Geometry check sheet. Reference: the model listing, model coordinates, mm. Face numbers are marked on the shaded views. A direction names the side the tool comes from. Coordinates: 2 decimals unless noted, no trailing zeros. Order: outer loops, then holes, each group sorted by start corner. A loop starts at its lowest first (then second) coordinate and runs counter-clockwise, first axis right, second up. Notation, with made-up numbers: (-29, 18) - (-16, 18) arc R16 ccw to (-16, 27) - close; hole circle Ø11 at (16, -1.5). An arc over 180 degrees is marked (long way). Return JSON: item names as keys, results as strings. Group by question number.
Item 1: Section check B-B on z = 32.5. Enter the section's corners in (x, y).
Item 2: Gauge pin test, flat ends, axial feed: pin 1 (0.9 mm diameter, centred on x = 0.5, y = 0.5, fed in from -Z); pin 2 (6 mm diameter, centred on x = 3, z = 18, fed in from +Y); pin 3 (3 mm diameter, centred on y = -0.5, z = 17, fed in from +X); pin 4 (3 mm diameter, centred on x = 2, y = 2, fed in from +Z). Record the tip position at first contact, or that the pin passes through.
Item 3: Scan lines: probe 1 along Z at (x, y) = (-2, -3.5); probe 2 along X at (y, z) = (0, 4); probe 3 along X at (y, z) = (1.5, 29). Record each from-to range of solid material in increasing order.
Item 4: Tool access check on the marked faces 1 and 2. Record the directions out of +Z, -Z, +X, -X, +Y, -Y that give a thin tool (end or side, any length) a straight path to the whole face; none if there is none.
Item 5: Section check A-A on y = 0. Enter the section's corners in (x, z).
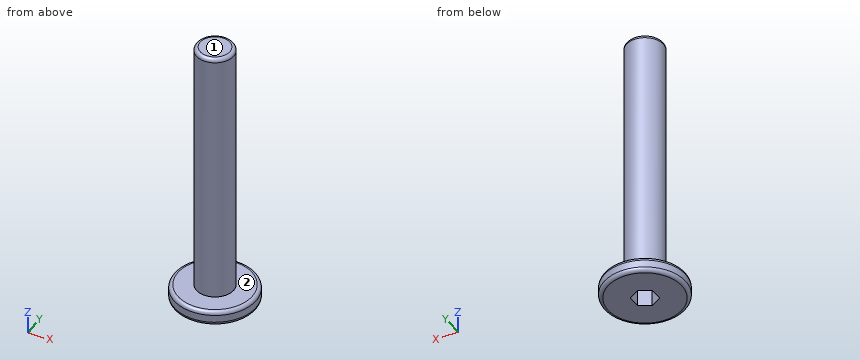
Autodesk Inventor part; units mm, degrees
ref_plane "YZ Plane" through (0, 0, 0) normal (1, 0, 0) x (0, 1, 0)
ref_plane "XZ Plane" through (0, 0, 0) normal (0, 1, 0) x (-1, 0, 0)
ref_plane "XY Plane" through (0, 0, 0) normal (0, 0, 1) x (1, 0, 0)
sketch "Sketch1" plane through (0, 0, 0) normal (1, 0, 0) x (0, 1, 0)
  line L0 (0, 0) -> (5.5, 0)
  line L1 (5.5, 0) -> (5.5, 2)
  line L2 (5.5, 2) -> (2.5, 2)
  line L3 (2.5, 2) -> (2.5, 37)
  line L4 (2.5, 37) -> (0, 37)
  line L5 (0, 37) -> (0, 0)
  dimension "d0" = 35
  dimension "d1" = 2
  dimension "d2" = 5.5
  dimension "d3" = 2.5
revolve "Revolution1" add sketch "Sketch1" angle 360 about axis through (0, 0, 37) along (0, 0, -1)
fillet "Fillet1" radius 0.5 3 edges at (0, -5.5, 0) (0, -5.5, 2) (0, -2.5, 37)
sketch "Sketch2" plane through (0, 0, 0) normal (0, 0, -1) x (-1, 0, 0)
  circle A0 centre (0, 0) radius 5
  line L0 (1.5, -0.866) -> (0, -1.7321)
  line L1 (0, -1.7321) -> (-1.5, -0.866)
  line L2 (-1.5, -0.866) -> (-1.5, 0.866)
  line L3 (-1.5, 0.866) -> (0, 1.7321)
  line L4 (0, 1.7321) -> (1.5, 0.866)
  line L5 (1.5, 0.866) -> (1.5, -0.866)
  dimension "d6" = 3
extrude "Extrusion1" cut sketch "Sketch2" against normal blind 3 contours L0 L1 L2 L3 L4 L5
thread "Thread1"
properties part number "M5x35 low profile screw"
Computed:
{
 "1": {"outline": "circle Ø5 at (0, 0)"},
 "2": {"pin 1": "stops at z = 3", "pin 2": "stops at y = 2.5", "pin 3": "stops at x = 2.5", "pin 4": "stops at z = 37"},
 "3": {"probe 1": "z = 0 to 2", "probe 2": "x = -2.5 to 2.5", "probe 3": "x = -2 to 2"},
 "4": {"face 1": "+Z, +X, -X, +Y, -Y", "face 2": "+Z"},
 "5": {"outline": "(-5.5, 0.5) arc R0.5 ccw to (-5, 0) - (-1.5, 0) - (-1.5, 3) - (1.5, 3) - (1.5, 0) - (5, 0) arc R0.5 ccw to (5.5, 0.5) - (5.5, 1.5) arc R0.5 ccw to (5, 2) - (2.5, 2) - (2.5, 36.5) arc R0.5 ccw to (2, 37) - (-2, 37) arc R0.5 ccw to (-2.5, 36.5) - (-2.5, 2) - (-5, 2) arc R0.5 ccw to (-5.5, 1.5) - close"}
}
